Solid Edge part; units mm, degrees
sketch "Sketch1" plane through (0, 0, 0) normal (0, 0, 1) x (1, 0, 0)
  line L0 (30, -25) -> (-30, -25)
  line L1 (-30, -25) -> (-30, 25)
  line L2 (-30, 25) -> (30, 25)
  line L3 (30, 25) -> (30, -25)
  dimension "D1" = 30
extrude "Protrusion1" add sketch "Sketch1" along normal blind 10
sketch "Sketch2" plane through (0, 0, 10) normal (0, 0, 1) x (1, 0, 0)
  line L0 (-23.5, 4.85) -> (-30, 4.85)
  line L1 (-30, 4.85) -> (-30, -4.85)
  line L2 (-30, -4.85) -> (-23.5, -4.85)
  arc A0 (-23.5, -4.85) -> (-23.5, 4.85) centre (-23.5, 0) ccw
  line L3 (23.5, 4.85) -> (30, 4.85)
  line L4 (30, -4.85) -> (30, 4.85)
  line L5 (23.5, -4.85) -> (30, -4.85)
  arc A1 (23.5, -4.85) -> (23.5, 4.85) centre (23.5, 0) cw
extrude "ProtrusiónExtruida_2" add sketch "Sketch2" along normal blind 19.5
sketch "Sketch3" plane through (-24.325, 0, 29.5) normal (0, 0, 1) x (1, 0, 0)
  circle A0 centre (0.825, 0) radius 2.15
  circle A1 centre (47.825, 0) radius 2.15
extrude "VaciadoExtruido_1" cut sketch "Sketch3" against normal blind 72.3664
sketch "Sketch4" plane through (0, 0, 0) normal (0, 0, -1) x (0, -1, 0)
  circle A0 centre (0, -23.5) radius 4
  circle A1 centre (0, 23.5) radius 4
extrude "VaciadoExtruido_2" cut sketch "Sketch4" against normal blind 6
sketch "Sketch5" plane through (0, 0, 10) normal (0, 0, 1) x (-1, 0, 0)
  line L0 (15.5, -25) -> (-15.5, -25)
  line L1 (-15.5, -25) -> (-15.5, 25)
  line L2 (-15.5, 25) -> (15.5, 25)
  line L3 (15.5, 25) -> (15.5, -25)
extrude "VaciadoExtruido_3" cut sketch "Sketch5" against normal blind 4.3
The listing builds one solid part. Answer for the finished solid, in the listing's coordinates (mm). A direction names the side the tool comes from. Give positions to 0.01 mm unless a question says otherwise; leave off trailing zeros. Write each loop counter-clockwise with the first axis right and the second up, starting at its lowest first coordinate (ties: lowest second). Pieces come first, ordered by that corner, then holes. Notation, with made-up numbers: (53, -8) - (57, -8) arc R15 cw to (57, 9) - close; hole circle Ø7 at (73.25, 85). An arc over 180 degrees is marked (long way). One line per question, with ' | ' between items. Start each with the question number.
1. Straight lines are drawn through the part: line 1 (X direction, y = 0, z = 1.5); line 2 (Y direction, x = -23.5, z = 1.3); line 3 (Z direction, x = 12.5, y = -8.5). For each, find the intervals that lie inside material, in ascending order.
2. For faces 1 (the face through (18.65, -0.11, 19.61)), 2 (the face through (-25, -2, 6)), 3 (the face through (-27, -4.85, 20)), 4 (the face through (-15.5, 0, 8)), 5 (the face through (27, 4.85, 20)), determine the directions among +Z, -Z, +X, -X, +Y, -Y from which every point of the face is accessible in a straight line to the end or side of a thin tool.
3. Section D-D, the plane z = 23.25 is taken. Determine the outline of the cut face in (x, y), then the cut area to 3 significant figures.
4. Determine the mould class of faces 6 (the face through (30, 0, 8)), 7 (the face through (19.534, 0.521, 2.958)), 8 (the face through (-27, 4.85, 20)) for opening direction Y: +Y half, -Y half, draft (parallel to the pull), parting line (faces both ways), or undercut.
5. Given P1, Ø7, axis at x = -23.5, y = -10.5, coming from the +Z side; P2, Ø5.5, axis at x = -23.5, y = 0, coming from the -Z side; P3, Ø2, axis at x = -25.5, z = 17.5, coming from the -Y side; P4, Ø10, axis at x = 10.5, z = 20, coming from the -Y side, each flat-ended and moving along its own axis, determine where each tip first touches the part or whether it passes through.
6. Section C-C, the plane y = 20.5 is taken. Determine the outline of the cut face in (x, z), then the cut area to 3 significant figures.
7. Section B-B, the plane y = 0 is taken. Determine the outline of the cut face in (x, z).
8. Section A-A, the plane z = 9.25 is taken. Determine the outline of the cut face in (x, y).
Result:
1) line 1: x = -30 to -27.5, -19.5 to 19.5, 27.5 to 30 | line 2: y = -25 to -4, 4 to 25 | line 3: z = 0 to 5.7
2) face 1: +Z | face 2: -Z | face 3: +Z, +X, -X, -Y | face 4: +Z, +Y, -Y | face 5: +Z, +X, -X, +Y
3) outline: (-30, -4.85) - (-23.5, -4.85) arc R4.85 ccw to (-23.5, 4.85) - (-30, 4.85) - close; (23.5, -4.85) - (30, -4.85) - (30, 4.85) - (23.5, 4.85) arc R4.85 ccw to start; hole circle Ø4.3 at (-23.5, 0); hole circle Ø4.3 at (23.5, 0) | area: 171 mm2
4) face 6: draft | face 7: undercut | face 8: +Y half
5) P1: stops at z = 10 | P2: stops at z = 6 | P3: stops at y = -4.85 | P4: passes through
6) outline: (-30, 0) - (30, 0) - (30, 10) - (15.5, 10) - (15.5, 5.7) - (-15.5, 5.7) - (-15.5, 10) - (-30, 10) - close | area: 467 mm2
7) outline: (-30, 0) - (-27.5, 0) - (-27.5, 6) - (-25.65, 6) - (-25.65, 29.5) - (-30, 29.5) - close; (-21.35, 6) - (-19.5, 6) - (-19.5, 0) - (19.5, 0) - (19.5, 6) - (21.35, 6) - (21.35, 29.5) - (18.65, 29.5) - (18.65, 10) - (15.5, 10) - (15.5, 5.7) - (-15.5, 5.7) - (-15.5, 10) - (-18.65, 10) - (-18.65, 29.5) - (-21.35, 29.5) - close; (25.65, 6) - (27.5, 6) - (27.5, 0) - (30, 0) - (30, 29.5) - (25.65, 29.5) - close
8) outline: (-30, -25) - (-15.5, -25) - (-15.5, 25) - (-30, 25) - close; (15.5, -25) - (30, -25) - (30, 25) - (15.5, 25) - close; hole circle Ø4.3 at (-23.5, 0); hole circle Ø4.3 at (23.5, 0)
